Verification items for the finished model (mm, model axes). Coordinates: 2 decimals unless noted, no trailing zeros. Loops run counter-clockwise (first coordinate to the right, second up) from the corner with the lowest first, then second, coordinate; pieces in that order, holes last.
Q1. Sectioned sample at D-D (x = -11.25). Enter the section's corners in (y, z).
Q2. Sectioned sample at C-C (y = 0.4). Count the separate pieces of the cut face and the enclosed holes in it, then the cut area to 3 significant figures.
Q3. Sectioned sample at B-B (z = 4.75). Enter the section's corners in (x, y), then the cut area to 4 significant figures.
Q4. Sectioned sample at A-A (x = 10). Enter the section's corners in (y, z).
Q5. Go/stop test with flat-tipped pins: P1, Ø0.6, axis at x = 0, y = 2, coming from the +Z side; P2, Ø5, axis at x = -10, z = 4.75, coming from the +Y side; P3, Ø1.4, axis at y = 2.5, z = 4, coming from the -X side. Record where each tip stops, or that it passes through.
Q6. Material ranges on probe 1 along X at (y, z) = (1.35, 6); probe 2 along Y at (x, z) = (0.75, -6); probe 3 along Z at (x, y) = (3.5, 1), recorded low to high.
```python
from build123d import *

# Parameters (mm, degrees)
SKETCH1_W           = 25.5
SKETCH1_H           = 15.5
SKETCH1_R           = 1.6
BOSS_EXTRUDE1_DEPTH = 1.5
SKETCH2_W           = 5.2
SKETCH2_H           = 3.8
BOSS_EXTRUDE2_DEPTH = 1.25
SKETCH3_R           = 0.5
CUT_EXTRUDE1_DEPTH  = 15.995832754
LPATTERN1_COUNT     = 10
LPATTERN1_PITCH     = 2.5


with BuildPart() as part:
    # Sketch1 → Boss-Extrude1 (new body)
    with BuildSketch(Plane(origin=(0, 0, 0), x_dir=(1, 0, 0), z_dir=(0, 1, 0))):
        Rectangle(SKETCH1_W, SKETCH1_H)
        with Locations(Location((-10, -4.75, 0), (0, 0, 270))):
            Circle(SKETCH1_R, mode=Mode.SUBTRACT)
        with Locations(Location((10, -4.75, 0), (0, 0, 270))):
            Circle(SKETCH1_R, mode=Mode.SUBTRACT)
    extrude(amount=BOSS_EXTRUDE1_DEPTH)

    # Sketch2 → Boss-Extrude2 (add)
    with BuildSketch(Plane(origin=(0, 1.5, 0), x_dir=(1, 0, 0), z_dir=(0, 1, 0))):
        with Locations((0, -3.65)):
            Rectangle(SKETCH2_W, SKETCH2_H)
    extrude(amount=BOSS_EXTRUDE2_DEPTH)

    # Sketch3 → Cut-Extrude1 (cut, through all)
    with BuildSketch(Plane(origin=(0, 1.5, 0), x_dir=(1, 0, 0), z_dir=(0, 1, 0))):
        with Locations(Location((-11.25, 6.25, 0), (0, 0, 270))):
            Circle(SKETCH3_R)
    cut_extrude1 = extrude(amount=-CUT_EXTRUDE1_DEPTH, mode=Mode.SUBTRACT)

    # LPattern1: Cut-Extrude1 ×10
    with Locations(*[(i * LPATTERN1_PITCH, 0, 0) for i in range(1, LPATTERN1_COUNT)]):
        add(cut_extrude1, mode=Mode.SUBTRACT)


solid = part.part
```
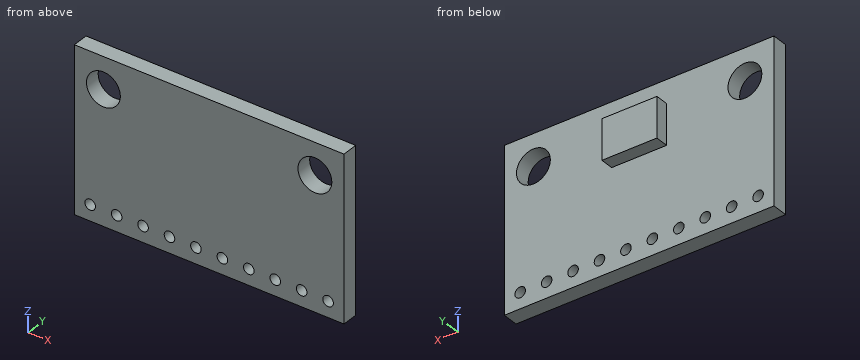
Geometry check:
1. outline: (0, -7.75) - (1.5, -7.75) - (1.5, -6.75) - (0, -6.75) - close; (0, -5.75) - (1.5, -5.75) - (1.5, 3.75) - (0, 3.75) - close; (0, 5.75) - (1.5, 5.75) - (1.5, 7.75) - (0, 7.75) - close
2. separate pieces: 1
2. enclosed holes: 12
2. area: 371 mm2
3. outline: (-12.75, 0) - (-11.6, 0) - (-11.6, 1.5) - (-12.75, 1.5) - close; (-8.4, 0) - (8.4, 0) - (8.4, 1.5) - (2.6, 1.5) - (2.6, 2.75) - (-2.6, 2.75) - (-2.6, 1.5) - (-8.4, 1.5) - close; (11.6, 0) - (12.75, 0) - (12.75, 1.5) - (11.6, 1.5) - close
3. area: 35.15 mm2
4. outline: (0, -7.75) - (1.5, -7.75) - (1.5, 3.15) - (0, 3.15) - close; (0, 6.35) - (1.5, 6.35) - (1.5, 7.75) - (0, 7.75) - close
5. P1: stops at z = 5.55
5. P2: stops at y = 1.5
5. P3: stops at x = -2.6
6. probe 1: x = -12.75 to -11, -9 to 9, 11 to 12.75
6. probe 2: y = 0 to 1.5
6. probe 3: z = -7.75 to -6.68, -5.82 to 7.75
